The listing builds one solid part. Answer for the finished solid, in the listing's coordinates (mm). Face numbers are marked on the shaded views. A direction names the side the tool comes from. Round coordinates to 2 decimals unless told otherwise and drop trailing zeros. Write each loop counter-clockwise with the first axis right and the second up, starting at its lowest first coordinate (ties: lowest second). Pieces come first, ordered by that corner, then holes. Notation, with made-up numbers: M 87.25,-3 L 134.25,-3 A17 cw 134.25,14 Z; hole C -8,36.5 d7. An arc over 180 degrees is marked long. One line per item, written item: value. Start each with the question number.
(1) Section C-C (y = 22.5) is taken. Determine the outline of the cut face in (x, z).
(2) Section B-B (z = 0) is taken. Determine the outline of the cut face in (x, y).
(3) Consider probe 1 along X at (y, z) = (36.5, 0); probe 2 along Y at (x, z) = (8, -10); probe 3 along Y at (x, z) = (3.5, -6). Determine where each line is inside the solid, lowest interval first.
(4) For a pull along Z with two mould halves and no side action, classify the marked faces 1, 2, 3 and 4 as released by +Z, released by -Z, zero draft, split by the parting line, or undercut.
(5) Section D-D (z = -9) is taken. Determine the outline of the cut face in (x, y).
(6) Section A-A (x = 0) is taken. Determine the outline of the cut face in (y, z).
(7) For the marked faces 5, 6, 7, 8 and 9, determine the directions among +Z, -Z, +X, -X, +Y, -Y from which every point of the face is accessible in a straight line to the end or side of a thin tool.
(8) Given P1, Ø5, axis at x = 0, z = -16, coming from the -Y side; P2, Ø8, axis at x = 0, z = 0, coming from the +Y side; P3, Ø4, axis at y = 17.5, z = 11.5, coming from the -X side; P4, Ø4, axis at y = 32, z = 10, coming from the +X side, each flat-ended and moving along its own axis, determine where each tip first touches the part or whether it passes through.
```python
from build123d import *

# Parameters (mm, degrees)
SKETCH_1_R          = 2.75
SKETCH_1_R_2        = 3.25
EXTRUDE_1_DEPTH     = 46.5
CUT_EXTRUDE_START   = -21.5
SKETCH_2_R          = 10.5
SKETCH_2_R_2        = 3.25
SKETCH_2_R_3        = 2.75
CUT_EXTRUDE_1_DEPTH = 21.5
SKETCH_4_R          = 5
CUT_EXTRUDE_3_DEPTH = 15
CUT_EXTRUDE_START_2 = -13
CUT_EXTRUDE_4_DEPTH = 13
FILLET_1_R          = 2.5
CUT_EXTRUDE_5_DEPTH = 5


with BuildPart() as part:
    # 草图1 → 凸台-拉伸1 (new body)
    with BuildSketch(Plane(origin=(0, 0, 0), x_dir=(1, 0, 0), z_dir=(0, 1, 0))):
        with BuildLine():
            Line((-6.112211857, 19.5), (5.859179501, 19.5))
            Line((5.859179501, 19.5), (11.054087418, 3.00371837))
            ThreePointArc((11.054087418, 3.00371837), (11.515865574, 0), (11.054087418, -3.00371837))
            Line((11.054087418, -3.00371837), (5.859179501, -19.5))
            Line((5.859179501, -19.5), (-6.112211857, -19.5))
            Line((-6.112211857, -19.5), (-11.127250475, -2.890493903))
            ThreePointArc((-11.127250475, -2.890493903), (-11.554108619, 0), (-11.127250475, 2.890493903))
            Line((-11.127250475, 2.890493903), (-6.112211857, 19.5))
        make_face()
        with Locations(Location((0, 16, 0), (0, 0, 90))):
            Circle(SKETCH_1_R, mode=Mode.SUBTRACT)
        with Locations(Location((0, 0, 0), (0, 0, 90))):
            Circle(SKETCH_1_R_2, mode=Mode.SUBTRACT)
        with Locations(Location((0, -16, 0), (0, 0, 90))):
            Circle(SKETCH_1_R, mode=Mode.SUBTRACT)
    extrude(amount=EXTRUDE_1_DEPTH)

    # 草图2 → 切除-拉伸1 (cut)
    # profile 1 of 3: a face of its own
    with BuildSketch(Plane(origin=(0, 46.5, 0), x_dir=(1, 0, 0), z_dir=(0, 1, 0)).offset(CUT_EXTRUDE_START)):
        with Locations(Location((0, 0, 0), (0, 0, 270))):
            Circle(SKETCH_2_R)
        with Locations(Location((0, 0, 0), (0, 0, 90))):
            Circle(SKETCH_2_R_2, mode=Mode.SUBTRACT)
    # profile 2 of 3: a face of its own
    with BuildSketch(Plane(origin=(0, 46.5, 0), x_dir=(1, 0, 0), z_dir=(0, 1, 0)).offset(CUT_EXTRUDE_START)):
        with BuildLine():
            Line((-6.112211857, 19.5), (-10.640039201, 4.504108324))
            ThreePointArc((-10.640039201, 4.504108324), (-0.240464733, 11.551606066), (10.443383029, 4.942992707))
            Line((10.443383029, 4.942992707), (5.859179501, 19.5))
            Line((5.859179501, 19.5), (-6.112211857, 19.5))
        make_face()
        with Locations(Location((0, 16, 0), (0, 0, 90))):
            Circle(SKETCH_2_R_3, mode=Mode.SUBTRACT)
    # profile 3 of 3: a face of its own
    with BuildSketch(Plane(origin=(0, 46.5, 0), x_dir=(1, 0, 0), z_dir=(0, 1, 0)).offset(CUT_EXTRUDE_START)):
        with BuildLine():
            Line((-6.112211857, -19.5), (5.859179501, -19.5))
            Line((5.859179501, -19.5), (10.443383029, -4.942992707))
            ThreePointArc((10.443383029, -4.942992707), (-0.240464733, -11.551606066), (-10.640039201, -4.504108324))
            Line((-10.640039201, -4.504108324), (-6.112211857, -19.5))
        make_face()
        with Locations(Location((0, -16, 0), (0, 0, 90))):
            Circle(SKETCH_2_R_3, mode=Mode.SUBTRACT)
    extrude(amount=CUT_EXTRUDE_1_DEPTH, mode=Mode.SUBTRACT)

    # 草图4 → 切除-拉伸3 (cut)
    with BuildSketch(Plane.XZ):
        with Locations(Location((0, 0, 0), (0, 0, 270))):
            Circle(SKETCH_4_R)
    extrude(amount=-CUT_EXTRUDE_3_DEPTH, mode=Mode.SUBTRACT)

    # 草图5 → 切除-拉伸4 (cut)
    with BuildSketch(Plane(origin=(0, 25, 0), x_dir=(1, 0, 0), z_dir=(0, 1, 0)).offset(CUT_EXTRUDE_START_2)):
        with BuildLine():
            Line((10.443383029, 4.942992707), (5.859179501, 19.5))
            Line((5.859179501, 19.5), (-6.112211857, 19.5))
            Line((-6.112211857, 19.5), (-10.640039201, 4.504108324))
            ThreePointArc((-10.640039201, 4.504108324), (-0.240464733, 11.551606066), (10.443383029, 4.942992707))
        make_face()
        with BuildLine():
            Line((-10.640039201, -4.504108324), (-6.112211857, -19.5))
            Line((-6.112211857, -19.5), (5.859179501, -19.5))
            Line((5.859179501, -19.5), (10.443383029, -4.942992707))
            ThreePointArc((10.443383029, -4.942992707), (-0.240464733, -11.551606066), (-10.640039201, -4.504108324))
        make_face()
    extrude(amount=CUT_EXTRUDE_4_DEPTH, mode=Mode.SUBTRACT)

    # 圆角1
    fillet_1_edges = [part.edges().sort_by_distance(p)[0] for p in [
        (5.859179501, 6, 19.5),
        (-6.112211857, 6, 19.5),
        (-6.112211857, 6, -19.5),
        (5.859179501, 6, -19.5),
    ]]
    fillet(fillet_1_edges, radius=FILLET_1_R)

    # 草图6 → 切除-拉伸5 (cut)
    with BuildSketch(Plane(origin=(0, 12, 0), x_dir=(1, 0, 0), z_dir=(0, 1, 0))):
        with BuildLine():
            Line((10.443383029, 4.942992707), (6.409986035, 17.750929593))
            ThreePointArc((6.409986035, 17.750929593), (5.504057643, 19.015852671), (4.025430574, 19.5))
            Line((4.025430574, 19.5), (-4.255583645, 19.5))
            ThreePointArc((-4.255583645, 19.5), (-5.74612739, 19.007057385), (-6.648869109, 17.722623476))
            Line((-6.648869109, 17.722623476), (-10.640039201, 4.504108324))
            ThreePointArc((-10.640039201, 4.504108324), (-0.240464733, 11.551606066), (10.443383029, 4.942992707))
        make_face()
        with BuildLine():
            Line((-10.640039201, -4.504108324), (-6.648869109, -17.722623476))
            ThreePointArc((-6.648869109, -17.722623476), (-5.74612739, -19.007057385), (-4.255583645, -19.5))
            Line((-4.255583645, -19.5), (4.025430574, -19.5))
            ThreePointArc((4.025430574, -19.5), (5.504057643, -19.015852671), (6.409986035, -17.750929593))
            Line((6.409986035, -17.750929593), (10.443383029, -4.942992707))
            ThreePointArc((10.443383029, -4.942992707), (-0.240464733, -11.551606066), (-10.640039201, -4.504108324))
        make_face()
    extrude(amount=-CUT_EXTRUDE_5_DEPTH, mode=Mode.SUBTRACT)


solid = part.part
```
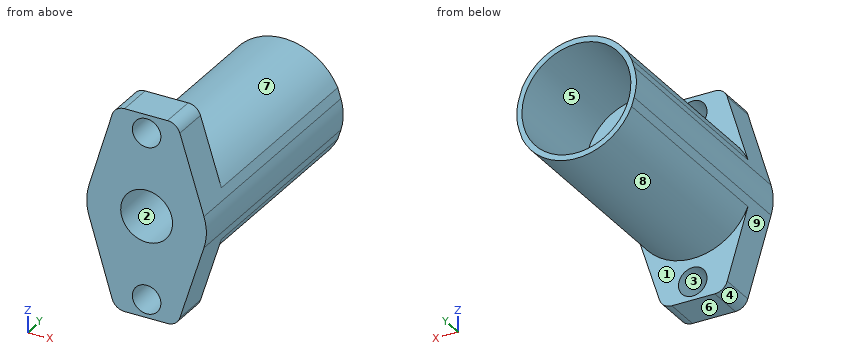
Recorded:
1. outline: M -11.13,-2.89 L -10.64,-4.5 A11.55 ccw 10.44,-4.94 L 11.05,-3 A10 ccw 11.05,3 L 10.44,4.94 A11.55 ccw -10.64,4.5 L -11.13,2.89 A10 ccw Z; hole C 0,0 d6.5
2. outline: M -11.55,0 L -5,0 L -5,15 L -3.25,15 L -3.25,25 L -10.5,25 L -10.5,46.5 L -11.55,46.5 Z; M 3.25,15 L 5,15 L 5,0 L 11.52,0 L 11.52,46.5 L 10.5,46.5 L 10.5,25 L 3.25,25 Z
3. probe 1: x = -11.55 to -10.5, 10.5 to 11.52
3. probe 2: y = 0 to 7
3. probe 3: y = 0 to 25
4. face 1: zero draft
4. face 2: undercut
4. face 3: undercut
4. face 4: released by -Z
5. outline: M -9.28,0 L 9.17,0 L 9.17,7 L 7.25,7 L 7.25,46.5 L 5.41,46.5 L 5.41,25 L -5.41,25 L -5.41,46.5 L -7.25,46.5 L -7.25,7 L -9.28,7 Z
6. outline: M 0,-19.5 L 7,-19.5 L 7,-18.75 L 0,-18.75 Z; M 0,-13.25 L 7,-13.25 L 7,-11.55 L 46.5,-11.55 L 46.5,-10.5 L 25,-10.5 L 25,-3.25 L 15,-3.25 L 15,-5 L 0,-5 Z; M 0,5 L 15,5 L 15,3.25 L 25,3.25 L 25,10.5 L 46.5,10.5 L 46.5,11.55 L 7,11.55 L 7,13.25 L 0,13.25 Z; M 0,18.75 L 7,18.75 L 7,19.5 L 0,19.5 Z
7. face 5: +Y
7. face 6: -Z, +X, -X, +Y, -Y
7. face 7: +Z, +Y
7. face 8: -Z, +Y
7. face 9: -Z, -X, +Y, -Y
8. P1: passes through
8. P2: stops at y = 25
8. P3: stops at x = -6.58
8. P4: stops at x = 8.34
